Can you work these out from the drawing? Everything is in mm from the part's minimum corner. A direction names the side the tool comes from. Coordinates: 2 decimals unless noted, no trailing zeros. Order: outer loops, then holes, each group sorted by start corner. A loop starts at its lowest first (then second) coordinate and runs counter-clockwise, first axis right, second up. Notation, with made-up numbers: (44, 53) - (88, 53) arc R21 cw to (88, 76) - close; hole circle Ø7 at (6.25, -36). An arc over 180 degrees is marked (long way). Use CSV: the item, a comma, the result in double quotes. Start each with the question number.
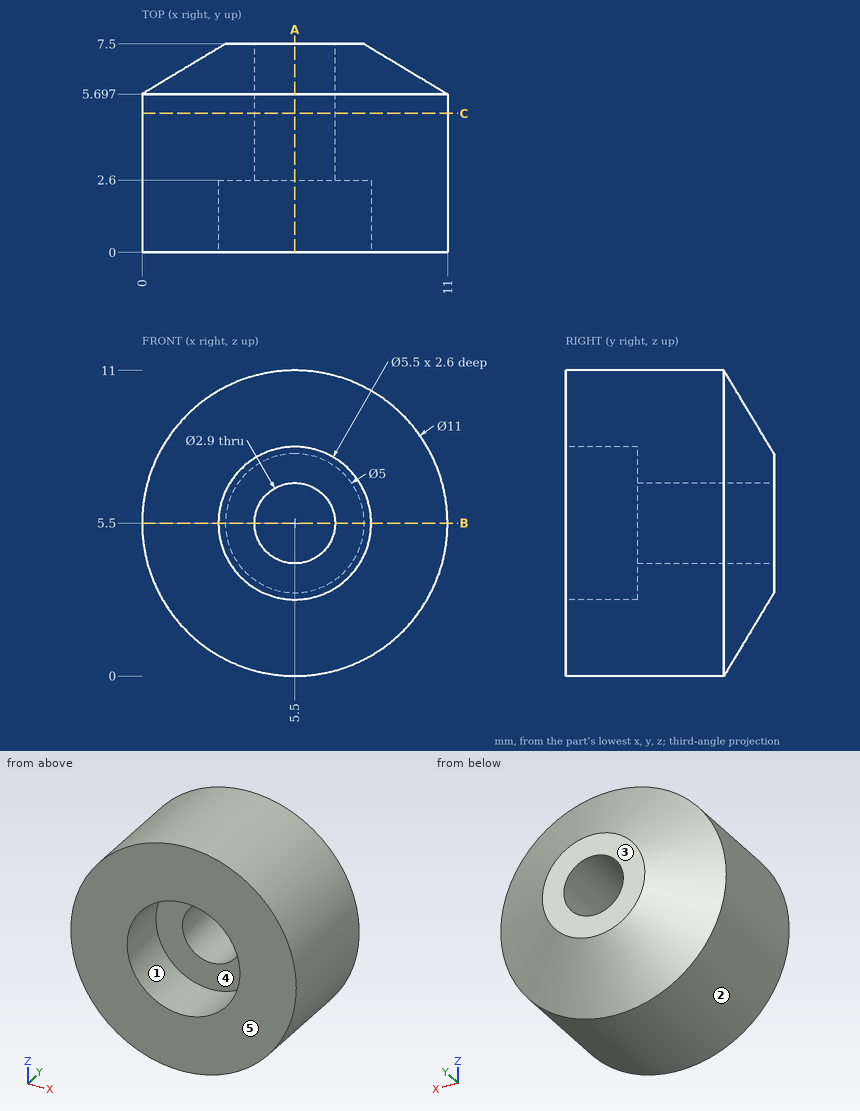
Item 1: Suppose I cut it at B-B on z = 5.5. Write out the boundary of the cut face in (x, y).
Item 2: For pin 1 Ø1.5 at (x, y) = (2, 5) entering from +Z; pin 2 Ø2.5 at (x, z) = (5.5, 5.5) entering from +Y; pin 3 Ø1 at (y, z) = (4, 6.5) entering from -X; pin 4 Ø1.5 at (y, z) = (5.5, 6.5) entering from +X, each with a flat end and sliding along its axis, tell me the tip position at first contact or that it passes through.
Item 3: Please list where these lines run through material, in increasing order: line 1 along X through (y, z) = (5.4, 5.5); line 2 along Z through (x, y) = (7, 1) (1 decimal). Write a range as from..to.
Item 4: Suppose I cut it at C-C on y = 5. Write out the boundary of the cut face in (x, z).
Item 5: For the marked faces 4 and 5, which set-ups out of +Z, -Z, +X, -X, +Y, -Y let a thin tool reach every point of the face, with its end or its side?
Item 6: We'd pull the mould along X, two halves only. Please class the marked faces 1, 2 and 3: released by +X, released by -X, zero draft, split by the parting line, or undercut.
Item 7: Suppose I cut it at A-A on x = 5.5. Write out the boundary of the cut face in (y, z).
Here are the results:
1,outline,"(0, 0) - (2.75, 0) - (2.75, 2.6) - (4.05, 2.6) - (4.05, 7.5) - (3, 7.5) - (0, 5.7) - close; (6.95, 2.6) - (8.25, 2.6) - (8.25, 0) - (11, 0) - (11, 5.7) - (8, 7.5) - (6.95, 7.5) - close"
2,pin 1,"z = 10.26"
2,pin 2,"through"
2,pin 3,"x = 0.02"
2,pin 4,"x = 10.99"
3,line 1,"0..4.05, 6.95..11"
3,line 2,"0.2..3.2, 7.8..10.8"
4,outline,"circle Ø11 at (5.5, 5.5); hole circle Ø2.9 at (5.5, 5.5)"
5,face 4,"-Y"
5,face 5,"+Z, -Z, +X, -X, -Y"
6,face 1,"undercut"
6,face 2,"split by the parting line"
6,face 3,"zero draft"
7,outline,"(0, 0) - (5.7, 0) - (7.5, 3) - (7.5, 4.05) - (2.6, 4.05) - (2.6, 2.75) - (0, 2.75) - close; (0, 8.25) - (2.6, 8.25) - (2.6, 6.95) - (7.5, 6.95) - (7.5, 8) - (5.7, 11) - (0, 11) - close"
